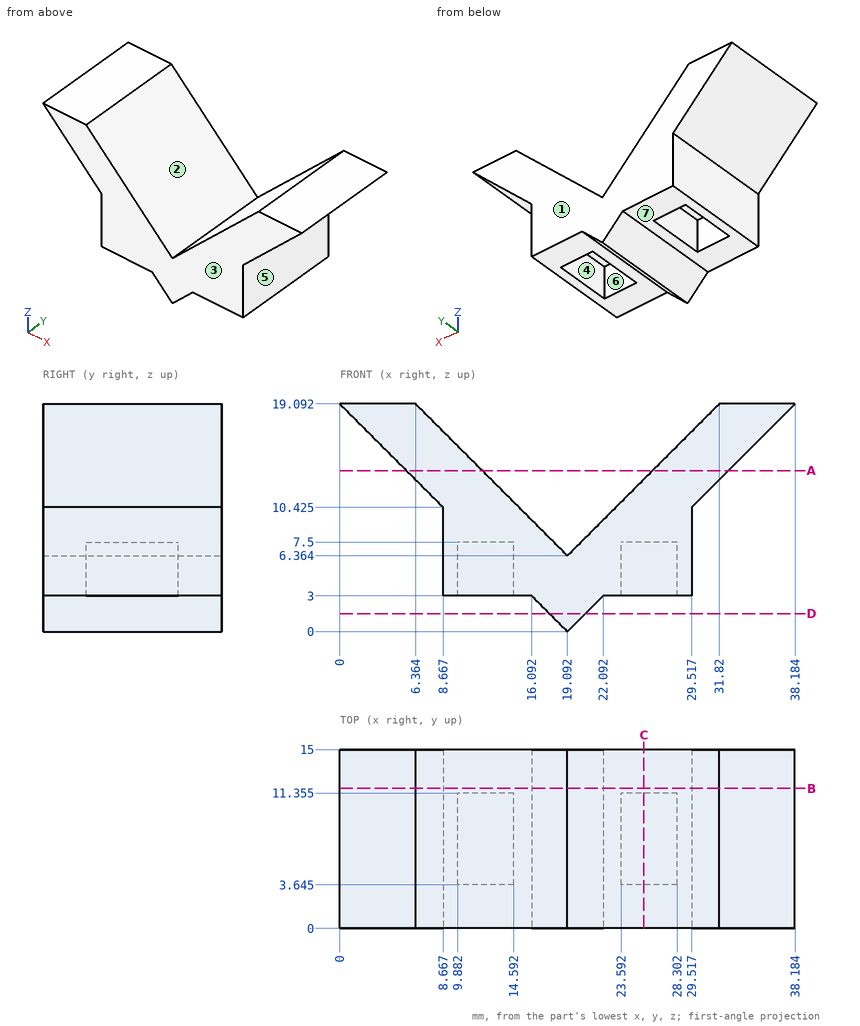
Verification items for this drawing (mm, ordinates from the low corner). A direction names the side the tool comes from. Coordinates: 2 decimals unless noted, no trailing zeros. Write each loop counter-clockwise with the first axis right and the second up, starting at its lowest first coordinate (ties: lowest second). Pieces come first, ordered by that corner, then holes. Notation, with made-up numbers: M 5.5,46 L 52.5,46 A25 cw 52.5,69 Z; hole C 50,37 d9. An arc over 180 degrees is marked long. Answer as CSV lines item,"result".
Q1. Go/stop test with flat-tipped pins: pin 1 (1.5 mm diameter, centred on x = 16, y = 7, fed in from +Z) (1 decimal); pin 2 (8 mm diameter, centred on y = 9.5, z = 8, fed in from +X); pin 3 (2.5 mm diameter, centred on x = 25, y = 7, fed in from -Z). Record where each tip stops, or that it passes through.
Check result:
pin 1,"z = 10.2"
pin 2,"x = 31.09"
pin 3,"z = 7.5"
Q2. Set-up check for the marked faces 5, 6 and 7: record each of +Z, -Z, +X, -X, +Y, -Y from which the full face is reachable in a straight line by a thin tool's end or side.
Check result:
face 5,"-Z, +X, +Y, -Y"
face 6,"-Z"
face 7,"-Z, -X, +Y, -Y"
Q3. Mould release check, pull along Y, two halves, no side actions. Record for the marked faces 1, 2, 3 and 4: released by +Y, released by -Y, zero draft, split by the parting line, or undercut.
Check result:
face 1,"released by +Y"
face 2,"zero draft"
face 3,"released by -Y"
face 4,"undercut"
Q4. Cross-section at B-B (y = 11.75). Record the boundary of the cut face in (x, z) (1 decimal).
Check result:
outline,"M 0,19.1 L 8.7,10.4 L 8.7,3 L 16.1,3 L 19.1,0 L 22.1,3 L 29.5,3 L 29.5,10.4 L 38.2,19.1 L 31.8,19.1 L 19.1,6.4 L 6.4,19.1 Z"
Q5. Cross-section at A-A (z = 13.5). Record the boundary of the cut face in (x, y) (1 decimal), then the cut area to 3 significant figures.
Check result:
outline,"M 5.6,0 L 12,0 L 12,15 L 5.6,15 Z; M 26.2,0 L 32.6,0 L 32.6,15 L 26.2,15 Z"
area,"191 mm^2"
Q6. Material ranges on probe 1 along X at (y, z) = (8, 4.75); probe 2 along Y at (x, z) = (27, 6) (1 decimal); probe 3 along X at (y, z) = (12, 4), recorded low to high. Write a range as from..to.
Check result:
probe 1,"8.67..9.88, 14.59..23.59, 28.3..29.52"
probe 2,"0..3.6, 11.4..15"
probe 3,"8.67..29.52"
Q7. Cross-section at D-D (z = 1.5). Record the boundary of the cut face in (x, y), then the cut area to 3 significant figures.
Check result:
outline,"M 17.59,0 L 20.59,0 L 20.59,15 L 17.59,15 Z"
area,"45.0 mm^2"
Q8. Cross-section at C-C (x = 25.5). Record the boundary of the cut face in (y, z) (1 decimal).
Check result:
outline,"M 0,3 L 3.6,3 L 3.6,7.5 L 11.4,7.5 L 11.4,3 L 15,3 L 15,12.8 L 0,12.8 Z"
